Autodesk Inventor part; units mm, degrees
ref_plane "YZ Plane" through (0, 0, 0) normal (1, 0, 0) x (0, 1, 0)
ref_plane "XZ Plane" through (0, 0, 0) normal (0, 1, 0) x (-1, 0, 0)
ref_plane "XY Plane" through (0, 0, 0) normal (0, 0, 1) x (1, 0, 0)
sketch "Sketch1" plane through (0, 0, 0) normal (0, 1, 0) x (-1, 0, 0)
  line L0 (0, 50) -> (0, 20) construction
  line L1 (0, -20) -> (0, -50) construction
  line L2 (-43.3013, 25) -> (-17.3205, 10) construction
  line L3 (18.0217, -8.6728) -> (44.0318, -23.6897) construction
  line L4 (-43.3013, -25) -> (-17.3205, -10) construction
  line L5 (17.3205, 10) -> (43.3013, 25) construction
  line L6 (-1.5, -19.9437) -> (-1.5, -49.9775)
  line L7 (1.5, -19.9437) -> (1.5, -49.9775)
  line L8 (-44.0318, -23.6897) -> (-18.0217, -8.6728)
  line L9 (-42.5318, -26.2878) -> (-16.5217, -11.2709)
  line L10 (-44.0318, 23.6897) -> (-18.0217, 8.6728)
  line L11 (-42.5318, 26.2878) -> (-16.5217, 11.2709)
  line L12 (-1.5, 49.9775) -> (-1.5, 19.9437)
  line L13 (1.5, 49.9775) -> (1.5, 19.9437)
  line L14 (16.5217, 11.2709) -> (42.5318, 26.2878)
  line L15 (18.0217, 8.6728) -> (44.0318, 23.6897)
  line L16 (17.3205, -10) -> (43.3013, -25)
  line L17 (18.6245, -7.2888) -> (44.7233, -22.3569)
  arc A0 (-1.5, -49.9775) -> (1.5, -49.9775) centre (0, 0) ccw
  arc A1 (-44.0318, -23.6897) -> (-42.5318, -26.2878) centre (0, 0) ccw
  arc A2 (-42.5318, 26.2878) -> (-44.0318, 23.6897) centre (0, 0) ccw
  arc A3 (1.5, 49.9775) -> (-1.5, 49.9775) centre (0, 0) ccw
  arc A4 (43.3013, -25) -> (44.7233, -22.3569) centre (0, 0) ccw
  arc A5 (44.0318, 23.6897) -> (42.5318, 26.2878) centre (0, 0) ccw
  arc A6 (16.5217, 11.2709) -> (1.5, 19.9437) centre (0, 0) ccw
  arc A7 (18.6245, -7.2888) -> (18.0217, 8.6728) centre (0, 0) ccw
  arc A8 (1.5, -19.9437) -> (17.3205, -10) centre (0, 0) ccw
  arc A9 (-16.5217, -11.2709) -> (-1.5, -19.9437) centre (0, 0) ccw
  arc A10 (-1.5, 19.9437) -> (-16.5217, 11.2709) centre (0, 0) ccw
  arc A11 (-18.0217, 8.6728) -> (-18.0217, -8.6728) centre (0, 0) ccw
  dimension "d8" = 1.5
  dimension "d9" = 1.5
  dimension "d10" = 1.5
  dimension "d11" = 1.5
  dimension "d12" = 1.5
  dimension "d13" = 1.5
  dimension "d14" = 1.5
  dimension "d15" = 1.5
  dimension "d16" = 1.5
  dimension "d17" = 1.5
  dimension "d18" = 1.5
  dimension "d19" = 1.5
extrude "Extrusion1" add sketch "Sketch1" along normal blind 30
fillet "Fillet1" radius 5 12 edges at (-43.3013, 30, 25) (-43.3013, 0, 25) (-44.0321, 30, -23.6891) (-44.0321, 0, -23.6891) (0, 30, 50) (0, 0, 50) (43.3013, 0, 25) (43.3013, 30, 25) (43.3013, 30, -25) (43.3013, 0, -25) (0, 30, -50) (0, 0, -50)
sketch "Sketch2" plane through (0, 30, 0) normal (0, 1, 0) x (1, 0, 0)
  arc A0 (1.5, 44.975) -> (-1.5, 44.975) centre (0, 0) ccw construction
  line L0 (-1.5, 44.975) -> (-1.5, 19.9437) construction
  arc A1 (-1.5, 19.9437) -> (-17.3205, 10) centre (0, 0) ccw construction
  line L1 (-17.3205, 10) -> (-38.9711, 22.5) construction
  arc A2 (-38.9711, 22.5) -> (-40.3844, 19.8519) centre (0, 0) ccw construction
  line L2 (-40.3844, 19.8519) -> (-18.6245, 7.2888) construction
  arc A3 (-18.6245, 7.2888) -> (-18.0217, -8.6728) centre (0, 0) ccw construction
  line L3 (-18.0217, -8.6728) -> (-39.6995, -21.1885) construction
  arc A4 (-39.6995, -21.1885) -> (-38.1995, -23.7865) centre (0, 0) ccw construction
  line L4 (-38.1995, -23.7865) -> (-16.5217, -11.2709) construction
  arc A5 (-16.5217, -11.2709) -> (-1.5, -19.9437) centre (0, 0) ccw construction
  line L5 (-1.5, -19.9437) -> (-1.5, -44.975) construction
  arc A6 (-1.5, -44.975) -> (1.5, -44.975) centre (0, 0) ccw construction
  line L6 (1.5, -44.975) -> (1.5, -19.9437) construction
  arc A7 (1.5, -19.9437) -> (16.5217, -11.2709) centre (0, 0) ccw construction
  line L7 (16.5217, -11.2709) -> (38.1995, -23.7865) construction
  arc A8 (38.1995, -23.7865) -> (39.6995, -21.1885) centre (0, 0) ccw construction
  line L8 (39.6995, -21.1885) -> (18.0217, -8.6728) construction
  arc A9 (18.0217, -8.6728) -> (18.0217, 8.6728) centre (0, 0) ccw construction
  line L9 (18.0217, 8.6728) -> (39.6995, 21.1885) construction
  arc A10 (39.6995, 21.1885) -> (38.1995, 23.7865) centre (0, 0) ccw construction
  line L10 (38.1995, 23.7865) -> (16.5217, 11.2709) construction
  arc A11 (16.5217, 11.2709) -> (1.5, 19.9437) centre (0, 0) ccw construction
  line L11 (1.5, 19.9437) -> (1.5, 44.975) construction
  circle A12 centre (0, 0) radius 1.5
  dimension "d23" = 3
extrude "Extrusion2" cut sketch "Sketch2" against normal blind 5
equation "\"d8\" = 0.5 * blade_width"
equation "\"d9\" = 0.5 * blade_width"
equation "\"d10\" = 0.5 * blade_width"
equation "\"d11\" = 0.5 * blade_width"
equation "\"d12\" = 0.5 * blade_width"
equation "\"d13\" = 0.5 * blade_width"
equation "\"d14\" = 0.5 * blade_width"
equation "\"d15\" = 0.5 * blade_width"
equation "\"d16\" = 0.5 * blade_width"
equation "\"d17\" = 0.5 * blade_width"
equation "\"d18\" = 0.5 * blade_width"
equation "\"d19\" = 0.5 * blade_width"
equation "\"d20\" = blade_height"
equation "\"blade_width\" = 3"
equation "\"blade_height\" = 30"
properties part number "sketch_for_propeller"
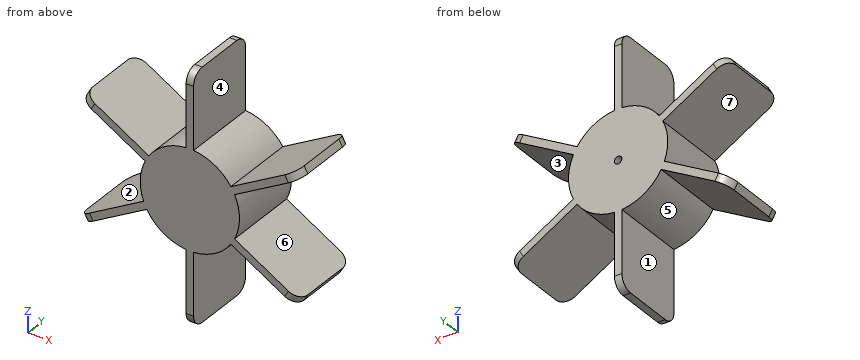
Could you check a few things on this model? Use its own coordinates, in mm. Face numbers are marked on the shaded views. A direction names the side the tool comes from. Coordinates: 2 decimals unless noted, no trailing zeros. Write each loop counter-clockwise with the first axis right and the second up, starting at its lowest first coordinate (ties: lowest second). Pieces come first, ordered by that corner, then holes. Notation, with made-up numbers: M 46,42 L 53,42 A27 cw 53,63 Z; hole C 60,13 d11. An arc over 180 degrees is marked long. Answer as CSV lines item,"result". Start each with the question number.
1) For P1, Ø15, axis at y = 22, z = 31, coming from the +X side; P2, Ø0.9, axis at x = 0, z = 0, coming from the +Y side; P3, Ø15, axis at y = 14, z = -30.5, coming from the -X side; P4, Ø10, axis at x = -11, z = 32, coming from the +Y side, each with a flat end and sliding along its axis, tell me the tip position at first contact or that it passes through.
2) I want a section at A-A, the plane x = -36. Please give me the cut outline in (y, z).
3) For the marked faces 4, 5, 6 and 7, which set-ups out of +Z, -Z, +X, -X, +Y, -Y let a thin tool reach every point of the face, with its end or its side?
4) I want a section at C-C, the plane y = 12. Please give me the cut outline in (x, z).
5) I want a section at B-B, the plane z = 0. Please give me the cut outline in (x, y).
6) Please list where these lines run through material, in increasing order: line 1 (X direction, y = 18, z = 21); line 2 (X direction, y = 3, z = -17.5); line 3 (X direction, y = 27, z = 0). Write a range as from..to.
7) I want a section at D-D, the plane z = -13.5. Please give me the cut outline in (x, y).
8) We'd pull the mould along X, two halves only. Please class the marked faces 1, 2 and 3: +X half, -X half, draft (parallel to the pull), parting line (faces both ways), or undercut.
Data:
1,P1,"stops at x = 44.03"
1,P2,"stops at y = 25"
1,P3,"stops at x = -44.4"
1,P4,"passes through"
2,outline,"M 0,-20.78 L 30,-20.78 L 30,-17.32 L 0,-17.32 Z; M 0,19.05 L 30,19.05 L 30,22.52 L 0,22.52 Z"
3,face 4,"+Z, +Y, -Y"
3,face 5,"-Z, +Y, -Y"
3,face 6,"+X, +Y, -Y"
3,face 7,"-X, +Y, -Y"
4,outline,"M -44.72,-22.36 A50.02 ccw -43.3,-25 L -17.32,-10 A20 ccw -1.5,-19.94 L -1.5,-49.98 A50 ccw 1.5,-49.98 L 1.5,-19.94 A20 ccw 16.52,-11.27 L 42.53,-26.29 A50.01 ccw 44.03,-23.69 L 18.02,-8.67 A20 ccw 18.02,8.67 L 44.03,23.69 A49.99 ccw 42.53,26.29 L 16.52,11.27 A20 ccw 1.5,19.94 L 1.5,49.98 A50 ccw -1.5,49.98 L -1.5,19.94 A20 ccw -16.52,11.27 L -42.53,26.29 A50.01 ccw -44.03,23.69 L -18.02,8.67 A20 ccw -18.62,-7.29 Z"
5,outline,"M -20,0 L 20,0 L 20,30 L 1.5,30 L 1.5,25 L -1.5,25 L -1.5,30 L -20,30 Z"
6,line 1,"x = -39.37..-33.37, -1.5..1.5, 33.37..39.37"
6,line 2,"x = -36.31..-30.31, -9.68..9.68, 27.31..33.31"
6,line 3,"x = -20..-1.5, 1.5..20"
7,outline,"M -29.38,0 L -23.38,0 L -23.38,30 L -29.38,30 Z; M -14.76,0 L 14.76,0 L 14.76,30 L -14.76,30 Z; M 20.38,0 L 26.38,0 L 26.38,30 L 20.38,30 Z"
8,face 1,"undercut"
8,face 2,"-X half"
8,face 3,"+X half"
